```python
from build123d import *

# Parameters (mm, degrees)
SKETCH1_R           = 32.5
BOSS_EXTRUDE1_DEPTH = 26
SKETCH2_R           = 5
BOSS_EXTRUDE2_DEPTH = 8
SKETCH3_R           = 2
CUT_EXTRUDE1_DEPTH  = 8
FILLET1_R           = 5


with BuildPart() as part:
    # Sketch1 → Boss-Extrude1 (new body)
    with BuildSketch(Plane(origin=(0, 0, 0), x_dir=(1, 0, 0), z_dir=(0, 1, 0))):
        with Locations(Location((0, 0, 0), (0, 0, 90))):
            Circle(SKETCH1_R)
    extrude(amount=BOSS_EXTRUDE1_DEPTH)

    # Sketch2 → Boss-Extrude2 (add)
    with BuildSketch(Plane(origin=(0, 26, 0), x_dir=(1, 0, 0), z_dir=(0, 1, 0))):
        with Locations(Location((0, 0, 0), (0, 0, 270))):
            Circle(SKETCH2_R)
    extrude(amount=BOSS_EXTRUDE2_DEPTH)

    # Sketch3 → Cut-Extrude1 (cut)
    with BuildSketch(Plane(origin=(0, 34, 0), x_dir=(1, 0, 0), z_dir=(0, 1, 0))):
        with Locations(Location((0, 0, 0), (0, 0, 270))):
            Circle(SKETCH3_R)
    extrude(amount=-CUT_EXTRUDE1_DEPTH, mode=Mode.SUBTRACT)

    # Fillet1
    fillet1_edges = [part.edges().sort_by_distance(p)[0] for p in [
        (0, 0, 32.5),
        (0, 26, 32.5),
    ]]
    fillet(fillet1_edges, radius=FILLET1_R)


solid = part.part
```
Check sheet for the modelled part. Datum: model origin and axes. Units: mm. A direction names the side the tool comes from. Coordinates: 2 decimals unless noted, no trailing zeros. Loops run counter-clockwise (first coordinate to the right, second up) from the corner with the lowest first, then second, coordinate; pieces in that order, holes last.
1) Sectioned sample at A-A (x = 0). Record the boundary of the cut face in (y, z).
2) Access from +Z, -Z, +X, -X, +Y, -Y to the whole of each face (thin tool, end or side, straight path). Record for faces 4 (the face through (-2, 30, 0)), 5 (the face through (0.1, 34, 2.2)).
3) Sectioned sample at B-B (y = 32.5). Record the boundary of the cut face in (x, z).
4) Material ranges on probe 1 along X at (y, z) = (30.25, 0); probe 2 along Y at (x, z) = (5, 7); probe 3 along X at (y, z) = (22, 4), recorded low to high.
5) Sectioned sample at C-C (z = 0). Record the boundary of the cut face in (x, y).
6) Release check for a two-part mould opening along Z. For faces 1 (the face through (0, 26, 0)), 2 (the face through (6, 26, 0)), 3 (the face through (-9.76, 12.89, -31)) record: released by +Z, released by -Z, zero draft, split by the parting line, or undercut.
7) Sectioned sample at D-D (y = 9). Record the boundary of the cut face in (x, z), and give its area (3 significant figures).
8) Gauge pin test, flat ends, axial feed: pin 1 (1.2 mm diameter, centred on x = 0, z = 1, fed in from +Y); pin 2 (1 mm diameter, centred on y = 14, z = 18.5, fed in from +X); pin 3 (4 mm diameter, centred on x = -11.5, y = 5.5, fed in from -Z). Record the tip position at first contact, or that the pin passes through.
Check sheet entries:
1. outline: (0, -27.5) arc R5 ccw to (5, -32.5) - (21, -32.5) arc R5 ccw to (26, -27.5) - (26, -5) - (34, -5) - (34, -2) - (26, -2) - (26, 2) - (34, 2) - (34, 5) - (26, 5) - (26, 27.5) arc R5 ccw to (21, 32.5) - (5, 32.5) arc R5 ccw to (0, 27.5) - close
2. face 4: +Y
2. face 5: +Z, -Z, +X, -X, +Y
3. outline: circle Ø10 at (0, 0); hole circle Ø4 at (0, 0)
4. probe 1: x = -5 to -2, 2 to 5
4. probe 2: y = 0 to 26
4. probe 3: x = -32.15 to 32.15
5. outline: (-32.5, 5) arc R5 ccw to (-27.5, 0) - (27.5, 0) arc R5 ccw to (32.5, 5) - (32.5, 21) arc R5 ccw to (27.5, 26) - (5, 26) - (5, 34) - (2, 34) - (2, 26) - (-2, 26) - (-2, 34) - (-5, 34) - (-5, 26) - (-27.5, 26) arc R5 ccw to (-32.5, 21) - close
6. face 1: undercut
6. face 2: zero draft
6. face 3: split by the parting line
7. outline: circle Ø65 at (0, 0)
7. area: 3,320 mm2
8. pin 1: stops at y = 26
8. pin 2: stops at x = 27.06
8. pin 3: stops at z = -31.08
